Build history of the part. All positions in model axes, mm. Give positions to 0.01 mm unless a question says otherwise; leave off trailing zeros. Order: outer loops, then holes, each group sorted by start corner. A loop starts at its lowest first (then second) coordinate and runs counter-clockwise, first axis right, second up. Notation, with made-up numbers: (3.5, 33.25) -> (18.5, 33.25) arc R24 cw to (18.5, 43.25) -> close; hole circle Ø10 at (82.25, -26.5). An arc over 180 degrees is marked (long way). Use a Markdown table: item, result. Add a question column.
```python
from build123d import *

# Parameters (mm, degrees)
SKETCH1_R               = 49.53
EXTRUDE1_DEPTH          = 1.5875
SKETCH2_R               = 2.06375
EXTRUDE2_DEPTH          = 10
MIRROR3_COPY_1_SKETCH_R = 2.06375
MIRROR3_COPY_1_DEPTH    = 10
CUT_EXTRUDE1_DEPTH      = 71.06398473
FILLET5_R               = 1.6
FILLET5_OF_MIRROR4_R    = 1.6
SKETCH4_R               = 1.18
CUT_EXTRUDE2_DEPTH      = 68.765197235
MIRROR6_COPY_1_SKETCH_R = 1.18
MIRROR6_COPY_1_DEPTH    = 68.765197235


with BuildPart() as part:
    # Sketch1 → Extrude1 (new body)
    with BuildSketch(Plane(origin=(0, 0, 0), x_dir=(1, 0, 0), z_dir=(0, 1, 0))):
        with Locations(Location((0, 0, 0), (0, 0, 270))):
            Circle(SKETCH1_R)
    extrude(amount=EXTRUDE1_DEPTH)

    # Sketch2 → Extrude2 (cut)
    with BuildSketch(Plane(origin=(0, 1.5875, 0), x_dir=(-1, 0, 0), z_dir=(0, 1, 0))):
        with Locations(Location((-26, -30, 0), (0, 0, 90))):
            Circle(SKETCH2_R)
    extrude2 = extrude(amount=-EXTRUDE2_DEPTH, mode=Mode.SUBTRACT)

    # Mirror1: Extrude2 across plane
    add(extrude2.mirror(Plane(origin=(0, 0, 0), x_dir=(0, 0, 1), z_dir=(1, 0, 0))), mode=Mode.SUBTRACT)

    # Mirror3: Extrude2 across plane
    add(extrude2.mirror(Plane.XY), mode=Mode.SUBTRACT)

    # Mirror3 copy 1 sketch → Mirror3 copy 1 (cut)
    with BuildSketch(Plane(origin=(0, 1.5875, 0), x_dir=(1, 0, 0), z_dir=(0, 1, 0))):
        with Locations(Location((-26, -30, 0), (0, 0, 90))):
            Circle(MIRROR3_COPY_1_SKETCH_R)
    extrude(amount=-MIRROR3_COPY_1_DEPTH, mode=Mode.SUBTRACT)

    # Sketch3 → Cut-Extrude1 (cut, through all)
    with BuildSketch(Plane(origin=(0, 1.5875, 0), x_dir=(1, 0, 0), z_dir=(0, 1, 0))):
        with BuildLine():
            Line((38.03, 0), (38.03, 17.8))
            Line((38.03, 17.8), (46.221000638, 17.8))
            ThreePointArc((46.221000638, 17.8), (49.53, 0), (46.221000638, -17.8))
            Line((46.221000638, -17.8), (38.03, -17.8))
            Line((38.03, -17.8), (38.03, 0))
        make_face()
    cut_extrude1 = extrude(amount=-CUT_EXTRUDE1_DEPTH, mode=Mode.SUBTRACT)

    # Fillet5
    fillet5_edges = [part.edges().sort_by_distance(p)[0] for p in [
        (38.03, 0.79375, 17.8),
        (38.03, 0.79375, -17.8),
    ]]
    fillet(fillet5_edges, radius=FILLET5_R)

    # Mirror4: Cut-Extrude1 across plane
    add(cut_extrude1.mirror(Plane(origin=(0, 0, 0), x_dir=(0, 0, 1), z_dir=(1, 0, 0))), mode=Mode.SUBTRACT)

    # Fillet5 of Mirror4
    fillet5_of_mirror4_edges = [part.edges().sort_by_distance(p)[0] for p in [
        (-38.03, 0.79375, 17.8),
        (-38.03, 0.79375, -17.8),
    ]]
    fillet(fillet5_of_mirror4_edges, radius=FILLET5_OF_MIRROR4_R)

    # Sketch4 → Cut-Extrude2 (cut, through all)
    with BuildSketch(Plane(origin=(0, 1.5875, 0), x_dir=(1, 0, 0), z_dir=(0, 1, 0))):
        with Locations(Location((6.731, -43.35, 0), (0, 0, 270))):
            Circle(SKETCH4_R)
    cut_extrude2 = extrude(amount=-CUT_EXTRUDE2_DEPTH, mode=Mode.SUBTRACT)

    # Mirror5: Cut-Extrude2 across plane
    add(cut_extrude2.mirror(Plane.XY), mode=Mode.SUBTRACT)

    # Mirror6: Cut-Extrude2 across plane
    add(cut_extrude2.mirror(Plane(origin=(0, 0, 0), x_dir=(0, 0, 1), z_dir=(1, 0, 0))), mode=Mode.SUBTRACT)

    # Mirror6 copy 1 sketch → Mirror6 copy 1 (cut, through all)
    with BuildSketch(Plane(origin=(0, 1.5875, 0), x_dir=(-1, 0, 0), z_dir=(0, 1, 0))):
        with Locations(Location((6.731, -43.35, 0), (0, 0, 270))):
            Circle(MIRROR6_COPY_1_SKETCH_R)
    extrude(amount=-MIRROR6_COPY_1_DEPTH, mode=Mode.SUBTRACT)


solid = part.part
```
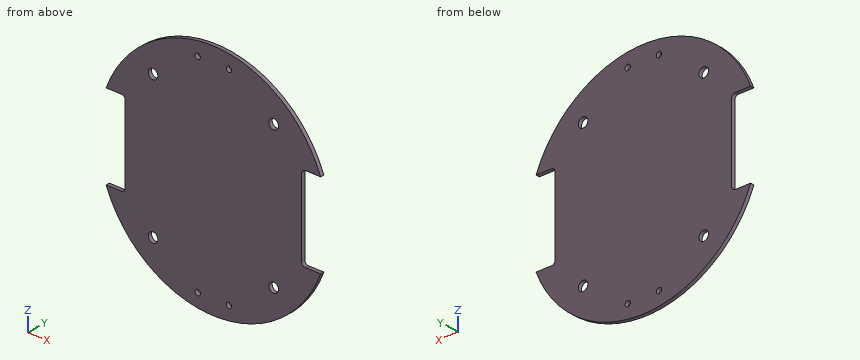
(1) Pin check, flat tips, straight feed: pin 1 Ø4.5 at (x, z) = (-26, -30) entering from -Y; pin 2 Ø0.8 at (x, y) = (41.5, 1) entering from -Z; pin 3 Ø0.8 at (y, z) = (1, 0) entering from -X; pin 4 Ø0.8 at (y, z) = (1, 2) entering from +X. Stop position of each tip, or through.
(2) Band-saw the part on D-D on z = -10. Give the cut face in (x, y).
(3) Band-saw the part on A-A on z = 43.35. Give the cut face in (x, y).
(4) Band-saw the part on B-B on x = 26. Give the cut face in (y, z).
(5) Band-saw the part on C-C on y = 0.85. State how many separate pieces and enclosed holes the cut face has, plus the area to 3 significant figures.
(6) Wall check: probe 1 along X at (y, z) = (1.1, 43.35); probe 2 along Z at (x, y) = (-25, 0.4); probe 3 along Z at (x, y) = (26.5, 1). Give the ranges that are in metal, low to high.
Response:
| question | item | result |
|---|---|---|
| 1 | pin 1 | stops at y = 0 |
| 1 | pin 2 | stops at z = -27.64 |
| 1 | pin 3 | stops at x = -38.03 |
| 1 | pin 4 | stops at x = 38.03 |
| 2 | outline | (-38.03, 0) -> (38.03, 0) -> (38.03, 1.59) -> (-38.03, 1.59) -> close |
| 3 | outline | (-23.96, 0) -> (-7.91, 0) -> (-7.91, 1.59) -> (-23.96, 1.59) -> close; (-5.55, 0) -> (5.55, 0) -> (5.55, 1.59) -> (-5.55, 1.59) -> close; (7.91, 0) -> (23.96, 0) -> (23.96, 1.59) -> (7.91, 1.59) -> close |
| 4 | outline | (0, -42.16) -> (1.59, -42.16) -> (1.59, -32.06) -> (0, -32.06) -> close; (0, -27.94) -> (1.59, -27.94) -> (1.59, 27.94) -> (0, 27.94) -> close; (0, 32.06) -> (1.59, 32.06) -> (1.59, 42.16) -> (0, 42.16) -> close |
| 5 | separate pieces | 1 |
| 5 | enclosed holes | 8 |
| 5 | area | 6,900 mm² |
| 6 | probe 1 | x = -23.96 to -7.91, -5.55 to 5.55, 7.91 to 23.96 |
| 6 | probe 2 | z = -42.76 to -31.81, -28.19 to 28.19, 31.81 to 42.76 |
| 6 | probe 3 | z = -41.84 to -32, -28 to 28, 32 to 41.84 |
